```python
from build123d import *

# Parameters (mm, degrees)
SKETCH2_R               = 7.5
SKETCH2_R_2             = 2.5
BOSS_EXTRUDE1_DEPTH     = 12
SKETCH4_R               = 6
SKETCH4_R_2             = 2.5
BOSS_EXTRUDE2_DEPTH     = 8
SKETCH7_R               = 4
BOSS_EXTRUDE3_DEPTH     = 8
BOSS_EXTRUDE3_2_DEPTH   = 8
BOSS_EXTRUDE3_3_DEPTH   = 8
BOSS_EXTRUDE4_DEPTH     = 2
SKETCH10_R              = 0.75
SKETCH10_R_2            = 2.5
CUT_EXTRUDE2_DEPTH      = 21
CUT_EXTRUDE2_DEPTH_BACK = 3
SKETCH12_R              = 57.284308747
CUT_EXTRUDE3_DEPTH      = 1
CUT_EXTRUDE3_DEPTH_BACK = 23
SKETCH15_R              = 1.6
CUT_EXTRUDE4_DEPTH      = 21
CUT_EXTRUDE4_DEPTH_BACK = 3
SKETCH13_R              = 1.6
BOSS_EXTRUDE5_DEPTH     = 2.5
SKETCH16_R              = 3.6
SKETCH16_R_2            = 1.6
BOSS_EXTRUDE6_DEPTH     = 21
CUT_EXTRUDE10_START     = -1
SKETCH19_R              = 3.6
SKETCH19_R_2            = 1.6
CUT_EXTRUDE10_DEPTH     = 4.5
CIRPATTERN1_COUNT       = 3


with BuildPart() as part:
    # Sketch2 → Boss-Extrude1 (new body)
    with BuildSketch(Plane(origin=(0, 0, 0), x_dir=(1, 0, 0), z_dir=(0, 1, 0))):
        Polygon((-37.230762114, -21.495190528), (37.230762114, -21.495190528), (0, 42.990381057), align=None)
        with Locations((0, 12.990381057)):
            Circle(SKETCH2_R, mode=Mode.SUBTRACT)
        with Locations((-11.25, -6.495190528)):
            Circle(SKETCH2_R, mode=Mode.SUBTRACT)
        with Locations((11.25, -6.495190528)):
            Circle(SKETCH2_R, mode=Mode.SUBTRACT)
        Circle(SKETCH2_R_2, mode=Mode.SUBTRACT)
    extrude(amount=BOSS_EXTRUDE1_DEPTH)

    # Sketch4 → Boss-Extrude2 (add)
    with BuildSketch(Plane.XZ):
        Polygon((-37.230762114, 21.495190528), (37.230762114, 21.495190528), (0, -42.990381057), align=None)
        with Locations((-11.25, 6.495190528)):
            Circle(SKETCH4_R, mode=Mode.SUBTRACT)
        with Locations((11.25, 6.495190528)):
            Circle(SKETCH4_R, mode=Mode.SUBTRACT)
        with Locations((0, -12.990381057)):
            Circle(SKETCH4_R, mode=Mode.SUBTRACT)
        Circle(SKETCH4_R_2, mode=Mode.SUBTRACT)
    extrude(amount=BOSS_EXTRUDE2_DEPTH)



with BuildPart() as body_2:
    # Sketch7 → Boss-Extrude3 (new body)
    with BuildSketch(Plane(origin=(0, -8, 0), x_dir=(1, 0, 0), z_dir=(0, 1, 0))):
        with Locations((0, 12.990381057)):
            Circle(SKETCH7_R)
    extrude(amount=BOSS_EXTRUDE3_DEPTH)


with BuildPart() as body_3:
    # Sketch7 → Boss-Extrude3 2 (new body)
    with BuildSketch(Plane(origin=(0, -8, 0), x_dir=(1, 0, 0), z_dir=(0, 1, 0))):
        with Locations((-11.25, -6.495190528)):
            Circle(SKETCH7_R)
    extrude(amount=BOSS_EXTRUDE3_2_DEPTH)


with BuildPart() as body_4:
    # Sketch7 → Boss-Extrude3 3 (new body)
    with BuildSketch(Plane(origin=(0, -8, 0), x_dir=(1, 0, 0), z_dir=(0, 1, 0))):
        with Locations((11.25, -6.495190528)):
            Circle(SKETCH7_R)
    extrude(amount=BOSS_EXTRUDE3_3_DEPTH)


with BuildPart() as part_1:
    add(part.part)

    add(body_2.part)  # Boss-Extrude4 merges body 2

    add(body_3.part)  # Boss-Extrude4 merges body 3

    add(body_4.part)  # Boss-Extrude4 merges body 4
    # Sketch9 → Boss-Extrude4 (add)
    with BuildSketch(Plane(origin=(0, -8, 0), x_dir=(1, 0, 0), z_dir=(0, 1, 0))):
        Polygon((0, 42.990381057), (-37.230762114, -21.495190528), (37.230762114, -21.495190528), align=None)
    extrude(amount=-BOSS_EXTRUDE4_DEPTH)

    # Sketch10 → Cut-Extrude2 (cut, two sides)
    with BuildSketch(Plane(origin=(0, -8, 0), x_dir=(1, 0, 0), z_dir=(0, 1, 0))) as cut_extrude2_sk:
        with Locations((-8.385990432, -2.3967214)):
            Circle(SKETCH10_R)
        with Locations((-12.668631437, -1.700663978)):
            Circle(SKETCH10_R)
        with Locations((-6.260007048, -6.17900967)):
            Circle(SKETCH10_R)
        with Locations((-7.891590133, -10.199388575)):
            Circle(SKETCH10_R)
        with Locations((-12.052124348, -11.430430799)):
            Circle(SKETCH10_R)
        with Locations((-15.608642568, -8.945136439)):
            Circle(SKETCH10_R)
        with Locations((-15.883014034, -4.614982838)):
            Circle(SKETCH10_R)
        with Locations((2.117373598, 8.46084145)):
            Circle(SKETCH10_R)
        with Locations((4.86149751, 11.821688644)):
            Circle(SKETCH10_R)
        with Locations((-2.22117582, 8.510829966)):
            Circle(SKETCH10_R)
        with Locations((-4.887134542, 11.934011819)):
            Circle(SKETCH10_R)
        with Locations((-3.872981274, 16.152661254)):
            Circle(SKETCH10_R)
        with Locations((0.057605887, 17.990049202)):
            Circle(SKETCH10_R)
        with Locations((3.944814641, 16.062585062)):
            Circle(SKETCH10_R)
        with Locations((6.268616834, -6.06412005)):
            Circle(SKETCH10_R)
        with Locations((7.807133926, -10.121024667)):
            Circle(SKETCH10_R)
        with Locations((8.481182868, -2.331820296)):
            Circle(SKETCH10_R)
        with Locations((12.778724676, -1.734623244)):
            Circle(SKETCH10_R)
        with Locations((15.925105622, -4.722230455)):
            Circle(SKETCH10_R)
        with Locations((15.55103668, -9.044912763)):
            Circle(SKETCH10_R)
        with Locations((11.938199393, -11.447602223)):
            Circle(SKETCH10_R)
        Circle(SKETCH10_R_2)
    extrude(amount=CUT_EXTRUDE2_DEPTH, mode=Mode.SUBTRACT)
    extrude(cut_extrude2_sk.sketch, amount=-CUT_EXTRUDE2_DEPTH_BACK, mode=Mode.SUBTRACT)

    # Sketch12 → Cut-Extrude3 (cut, two sides)
    with BuildSketch(Plane(origin=(0, 12, 0), x_dir=(1, 0, 0), z_dir=(0, 1, 0))) as cut_extrude3_sk:
        Circle(SKETCH12_R)
        with BuildLine():
            Line((-12.990381057, 20.490381057), (-24.240381057, 1.004809472))
            ThreePointArc((-24.240381057, 1.004809472), (-24.240381057, -13.995190528), (-11.25, -21.495190528))
            Line((-11.25, -21.495190528), (11.25, -21.495190528))
            ThreePointArc((11.25, -21.495190528), (24.240381057, -13.995190528), (24.240381057, 1.004809472))
            Line((24.240381057, 1.004809472), (12.990381057, 20.490381057))
            ThreePointArc((12.990381057, 20.490381057), (0, 27.990381057), (-12.990381057, 20.490381057))
        make_face(mode=Mode.SUBTRACT)
    extrude(amount=CUT_EXTRUDE3_DEPTH, mode=Mode.SUBTRACT)
    extrude(cut_extrude3_sk.sketch, amount=-CUT_EXTRUDE3_DEPTH_BACK, mode=Mode.SUBTRACT)

    # Sketch15 → Cut-Extrude4 (cut, two sides)
    with BuildSketch(Plane(origin=(0, -8, 0), x_dir=(1, 0, 0), z_dir=(0, 1, 0))) as cut_extrude4_sk:
        with Locations((0, 12.990381057)):
            Circle(SKETCH15_R)
        with Locations((-11.25, -6.495190528)):
            Circle(SKETCH15_R)
        with Locations((11.25, -6.495190528)):
            Circle(SKETCH15_R)
    extrude(amount=CUT_EXTRUDE4_DEPTH, mode=Mode.SUBTRACT)
    extrude(cut_extrude4_sk.sketch, amount=-CUT_EXTRUDE4_DEPTH_BACK, mode=Mode.SUBTRACT)

    # Sketch13 → Boss-Extrude5 (add)
    with BuildSketch(Plane(origin=(0, 12, 0), x_dir=(1, 0, 0), z_dir=(0, 1, 0))):
        with BuildLine():
            Line((-12.990381057, 20.490381057), (-24.240381057, 1.004809472))
            ThreePointArc((-24.240381057, 1.004809472), (-24.240381057, -13.995190528), (-11.25, -21.495190528))
            Line((-11.25, -21.495190528), (11.25, -21.495190528))
            ThreePointArc((11.25, -21.495190528), (24.240381057, -13.995190528), (24.240381057, 1.004809472))
            Line((24.240381057, 1.004809472), (12.990381057, 20.490381057))
            ThreePointArc((12.990381057, 20.490381057), (0, 27.990381057), (-12.990381057, 20.490381057))
        make_face()
        with BuildLine():
            ThreePointArc((11.258330249, 19.490381057), (0, 25.990381057), (-11.258330249, 19.490381057))
            Line((-11.258330249, 19.490381057), (-22.508330249, 0.004809472))
            ThreePointArc((-22.508330249, 0.004809472), (-22.508330249, -12.995190528), (-11.25, -19.495190528))
            Line((-11.25, -19.495190528), (11.25, -19.495190528))
            ThreePointArc((11.25, -19.495190528), (22.508330249, -12.995190528), (22.508330249, 0.004809472))
            Line((22.508330249, 0.004809472), (11.258330249, 19.490381057))
        make_face(mode=Mode.SUBTRACT)
        with Locations((0, -13.495190528)):
            Circle(SKETCH13_R)
        with Locations((11.687177826, 6.747595264)):
            Circle(SKETCH13_R)
        with Locations((-11.687177826, 6.747595264)):
            Circle(SKETCH13_R)
    extrude(amount=BOSS_EXTRUDE5_DEPTH)

    # Sketch16 → Boss-Extrude6 (add)
    with BuildSketch(Plane(origin=(0, 14.5, 0), x_dir=(1, 0, 0), z_dir=(0, 1, 0))):
        with Locations((-20.001021703, 11.547595264)):
            Circle(SKETCH16_R)
        with Locations((-20.001021703, 11.547595264)):
            Circle(SKETCH16_R_2, mode=Mode.SUBTRACT)
        with Locations((20.001021703, 11.547595264)):
            Circle(SKETCH16_R)
        with Locations((20.001021703, 11.547595264)):
            Circle(SKETCH16_R_2, mode=Mode.SUBTRACT)
        with Locations((0, -23.095190528)):
            Circle(SKETCH16_R)
        with Locations((0, -23.095190528)):
            Circle(SKETCH16_R_2, mode=Mode.SUBTRACT)
    extrude(amount=-BOSS_EXTRUDE6_DEPTH)

    # Sketch19 → Cut-Extrude10 (cut)
    with BuildSketch(Plane(origin=(0, -10, 0), x_dir=(1, 0, 0), z_dir=(0, 1, 0)).offset(CUT_EXTRUDE10_START)):
        with Locations((20.001021703, 11.547595264)):
            Circle(SKETCH19_R)
        with Locations((20.001021703, 11.547595264)):
            Circle(SKETCH19_R_2, mode=Mode.SUBTRACT)
    cut_extrude10 = extrude(amount=CUT_EXTRUDE10_DEPTH, mode=Mode.SUBTRACT)

    # CirPattern1: Cut-Extrude10 ×3 about axis
    cirpattern1_axis = Axis((0, 0, 0), (0, 1, 0))
    for i in range(1, CIRPATTERN1_COUNT):
        add(cut_extrude10.rotate(cirpattern1_axis, i * 360 / CIRPATTERN1_COUNT), mode=Mode.SUBTRACT)


solid = part_1.part
```
Source: CAD feature listing. Evaluate the final solid. Frame: model axes, mm. A direction names the side the tool comes from. Coordinates: 2 decimals unless noted, no trailing zeros. Write each loop counter-clockwise with the first axis right and the second up, starting at its lowest first coordinate (ties: lowest second). Pieces come first, ordered by that corner, then holes. Notation, with made-up numbers: (78, -5.5) - (137, -5.5) arc R12 ccw to (137, -0.5) - close; hole circle Ø11 at (-12.75, 80). An arc over 180 degrees is marked (long way). Answer as a JSON object with one key per item and string values.
Q1. Section query C-C, the plane y = 6.25. Output: boundary loops of the cut face in (x, z).
Ans:
{"outline": "(-24.24, -1) - (-20.23, -7.95) arc R3.6 ccw (long way) to (-17, -13.54) - (-12.99, -20.49) arc R15 ccw to (12.99, -20.49) - (17, -13.54) arc R3.6 ccw (long way) to (20.23, -7.95) - (24.24, -1) arc R15 ccw to (11.25, 21.5) - (3.22, 21.5) arc R3.6 ccw (long way) to (-3.22, 21.5) - (-11.25, 21.5) arc R15 ccw to start; hole circle Ø3.2 at (-20, -11.55); hole circle Ø15 at (-11.25, 6.5); hole circle Ø15 at (0, -12.99); hole circle Ø5 at (0, 0); hole circle Ø3.2 at (0, 23.1); hole circle Ø15 at (11.25, 6.5); hole circle Ø3.2 at (20, -11.55)"}
Q2. Draft query along Z for faces 1 (the cylindrical face through (7.254, -4.056, 6.319)), 2 (the cylindrical face through (-3.16, -8.99, -16.38)), 3 (the cylindrical face through (0.22, 2.08, -27.99)), 4 (the cylindrical face through (-24.35, 2.08, 13.8)). Return one class per face: released by +Z, released by -Z, zero draft, split by the parting line, or undercut.
Ans:
{"face 1": "undercut", "face 2": "undercut", "face 3": "released by -Z", "face 4": "split by the parting line"}
Q3. First-contact query: pin 1 Ø2.5 at (x, z) = (0.06, -17.99) entering from +Y; pin 2 Ø1.4 at (x, z) = (3.94, -16.06) entering from -Y; pin 3 Ø2 at (y, z) = (-5.5, -18.5) entering from +X; pin 4 Ø2 at (x, y) = (-5.5, 4.5) entering from -Z. Flat tips, straight axial feed; report the tip coordinate or a pass-through.
Ans:
{"pin 1": "stops at y = 0", "pin 2": "passes through", "pin 3": "stops at x = 14.72", "pin 4": "stops at z = -27.3"}
Q4. Section query A-A, the plane y = -3. State how many separate pieces and enclosed holes the cut face has, plus the area to 3 significant figures.
Ans:
{"separate pieces": "4", "enclosed holes": "10", "area": "1,780 mm2"}
Q5. Material intervals for line 1 (X direction, y = 4, z = 1.5); line 2 (X direction, y = -4, z = 23); line 3 (X direction, y = 2.5, z = 8.5), sorted ascending. Write a range as [from, to].
Ans:
{"line 1": "x = [-25.39, -16.84], [-5.66, -2], [2, 5.66], [16.84, 25.39]", "line 2": "x = [-3.6, -1.6], [1.6, 3.6]", "line 3": "x = [-26.12, -18.48], [-4.02, 4.02], [18.48, 26.12]"}
Q6. Set-up query: faces 5 (the cylindrical face through (0.19, 13.23, -25.99)), 6 (the cylindrical face through (2.81, -8.99, -8.17)). Return all of +Z, -Z, +X, -X, +Y, -Y with unobstructed straight access to the full face (end or side cutting, diameter ignored); none if empty.
Ans:
{"face 5": "+Y", "face 6": "+Y, -Y"}
